Geometry check sheet. Reference: the model listing, model coordinates, mm. Round coordinates to 2 decimals unless told otherwise and drop trailing zeros. Write each loop counter-clockwise with the first axis right and the second up, starting at its lowest first coordinate (ties: lowest second). Pieces come first, ordered by that corner, then holes. Notation, with made-up numbers: (5.25, 47) -> (11.25, 47) arc R19 cw to (11.25, 67) -> close; hole circle Ø11 at (-8.75, 27). An arc over 180 degrees is marked (long way). One line per question, with ' | ' between items.
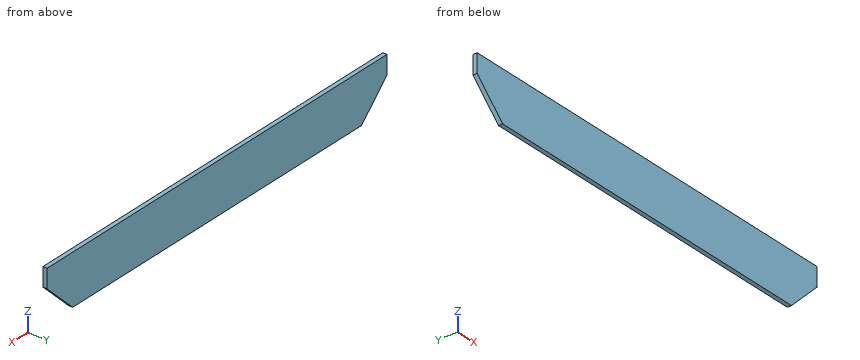
```python
from build123d import *

# Parameters (mm, degrees)
F0_W     = 170
F0_H     = 15
F1_DEPTH = 2


# Not quite as in the source:
# - a feature names something its author has since deleted; it is built from what else it names


with BuildPart() as f1:
    # F0 (on Front) → F1 (new body)
    with BuildSketch(Plane.XZ):
        Rectangle(F0_W, F0_H)
        Polygon((-100, 7.5), (-85, -7.5), (-85, 7.5), align=None)
        Polygon((85, 7.5), (85, -7.5), (100, 7.5), align=None)
        Polygon((-85, 7.5), (85, 7.5), (100, 7.5), (100, 16.5), (-100, 16.5), (-100, 7.5), align=None)
    extrude(amount=F1_DEPTH)


solid = f1.part
```
(1) Sectioned sample at A-A on y = -1.5. Record the cut outline in (x, z), then the cut area to 4 significant figures.
Resolved:
outline: (-100, 7.5) -> (-85, -7.5) -> (85, -7.5) -> (100, 7.5) -> (100, 16.5) -> (-100, 16.5) -> close | area: 4,575 mm2
(2) Material ranges on line 1 (X direction, y = -0.85, z = 1.5); line 2 (X direction, y = -1.6, z = -1.5), recorded low to high.
Resolved:
line 1: x = -94 to 94 | line 2: x = -91 to 91
(3) Go/stop test with flat-tipped pins: pin 1 (1 mm diameter, centred on x = -9.5, z = 10, fed in from +Y); pin 2 (1 mm diameter, centred on y = -1.5, z = -1.5, fed in from -X). Record where each tip stops, or that it passes through.
Resolved:
pin 1: stops at y = 0 | pin 2: stops at x = -91.5
(4) Sectioned sample at B-B on z = -1.5. Record the cut outline in (x, y), then the cut area to 3 significant figures.
Resolved:
outline: (-91, -2) -> (91, -2) -> (91, 0) -> (-91, 0) -> close | area: 364 mm2
